The listing builds one solid part. Answer for the finished solid, in the listing's coordinates (mm). Face numbers are marked on the shaded views. A direction names the side the tool comes from. Round coordinates to 2 decimals unless told otherwise and drop trailing zeros. Write each loop counter-clockwise with the first axis right and the second up, starting at its lowest first coordinate (ties: lowest second). Pieces come first, ordered by that corner, then holes. Notation, with made-up numbers: (65.25, -25) - (124.25, -25) arc R25 ccw to (124.25, 14) - close; hole circle Ø4 at (25.25, -28.5). An arc over 180 degrees is marked (long way). Use a Markdown table: item, result. Add a question column.
1) Determine the mould class of the marked faces 1, 2, 3 and 4 for opening direction X: +X half, -X half, draft (parallel to the pull), parting line (faces both ways), or undercut.
2) Find the intervals of material crossed by probe 1 along X at (y, z) = (15.25, 0); probe 2 along X at (y, z) = (21, -7.5); probe 3 along Z at (x, y) = (-8.5, 3.25), in increasing order. Write a range as from..to.
3) A cutting plane is placed at B-B (y = 11). Give the vertices of the cut face in (x, z), then the cut area to 3 significant figures.
4) A cutting plane is placed at D-D (x = 0). Give the vertices of the cut face in (y, z), then the cut area to 3 significant figures.
5) A cutting plane is placed at A-A (x = -15.05). Give the vertices of the cut face in (y, z).
6) Each of these flat-tipped pins is pushed along its axis until it touches: P1, Ø2, axis at x = 19.5, y = 6, coming from the -Z side; P2, Ø3.5, axis at y = 5, z = -18, coming from the +X side; P3, Ø4, axis at x = 43.53, z = -15, coming from the +Y side. Where does it stop, or does it pass through?
7) A tool of negligible diameter and unlimited length cuts with its end or side. For the marked faces 5, 6 and 7, from which of +Z, -Z, +X, -X, +Y, -Y can it reach the whole face along a straight path? Write none if from no direction.
8) A cutting plane is placed at C-C (y = 6). Give the vertices of the cut face in (x, z).
```python
from build123d import *

# Parameters (mm, degrees)
BOSS_EXTRUDE1_DEPTH             = 25
SKETCH2_R                       = 1.55
CUT_EXTRUDE1_DEPTH              = 22.5
BOSS_EXTRUDE2_REACH             = 65.436
BOSS_EXTRUDE2_DIRECTION_2_DEPTH = 30
CUT_EXTRUDE2_REACH              = 80.642
CUT_EXTRUDE2_END_RADIUS         = 17.5
SKETCH7_R                       = 1.55
SKETCH9_R                       = 2.05
CUT_EXTRUDE3_DEPTH              = 35.1
BOSS_EXTRUDE5_REACH             = 63.632


with BuildPart() as part:
    # Sketch1 → Boss-Extrude1 (new, symmetric)
    with BuildSketch(Plane.XY):
        with BuildLine():
            Line((-17.55, 22.5), (-17.55, 0))
            Line((-17.55, 0), (17.55, 0))
            Line((17.55, 0), (17.55, 22.5))
            Line((17.55, 22.5), (12.55, 22.5))
            ThreePointArc((12.55, 22.5), (0, 9.95), (-12.55, 22.5))
            Line((-12.55, 22.5), (-17.55, 22.5))
        make_face()
    extrude(amount=BOSS_EXTRUDE1_DEPTH, both=True)

    # Sketch2 → Cut-Extrude1 (cut)
    with BuildSketch(Plane(origin=(0, 22.5, 0), x_dir=(1, 0, 0), z_dir=(0, 1, 0))):
        with Locations(Location((-15.05, 0, 0), (0, 0, 270))):
            Circle(SKETCH2_R)
        with Locations(Location((15.05, 0, 0), (0, 0, 270))):
            Circle(SKETCH2_R)
    extrude(amount=-CUT_EXTRUDE1_DEPTH, mode=Mode.SUBTRACT)

    # Boss-Extrude2: up to this plane
    boss_extrude2_end = Plane(origin=(17.55, 0, 25), z_dir=(-1, 0, 0))
    # Sketch5 → Boss-Extrude2 (add, up to the surface)
    with BuildSketch(Plane(origin=(26.152881057, 0, -15.099372918), x_dir=(-0.5000000000000013, 0, -0.8660254037844379), z_dir=(0.8660254037844379, 0, -0.5000000000000013)), mode=Mode.PRIVATE) as boss_extrude2_sk1:
        with BuildLine():
            Line((-26.275, 22.5), (-21.325, 22.5))
            ThreePointArc((-21.325, 22.5), (-8.775, 9.95), (3.775, 22.5))
            Line((3.775, 22.5), (8.725, 22.5))
            ThreePointArc((8.725, 22.5), (-8.775, 5), (-26.275, 22.5))
        make_face()
    boss_extrude2_tool1 = split(extrude(boss_extrude2_sk1.sketch, amount=-BOSS_EXTRUDE2_REACH, mode=Mode.PRIVATE), bisect_by=boss_extrude2_end, keep=Keep.BOTH, mode=Mode.PRIVATE)
    add(boss_extrude2_tool1.solids().sort_by_distance((38.052881, 22.108688, 5.512032))[0])

    # Sketch5 → Boss-Extrude2 direction 2 (add)
    with BuildSketch(Plane(origin=(26.152881057, 0, -15.099372918), x_dir=(-0.5000000000000013, 0, -0.8660254037844379), z_dir=(0.8660254037844379, 0, -0.5000000000000013))):
        with BuildLine():
            Line((-26.275, 22.5), (-21.325, 22.5))
            ThreePointArc((-21.325, 22.5), (-8.775, 9.95), (3.775, 22.5))
            Line((3.775, 22.5), (8.725, 22.5))
            ThreePointArc((8.725, 22.5), (-8.775, 5), (-26.275, 22.5))
        make_face()
    extrude(amount=BOSS_EXTRUDE2_DIRECTION_2_DEPTH)

    # Cut-Extrude2: up to this cylinder (the profile starts inside it)
    cut_extrude2_end = Plane(origin=(43.530762028, 22.5, -14.999999951), z_dir=(-0.8660254037844379, 0, 0.5000000000000013)) * Cylinder(CUT_EXTRUDE2_END_RADIUS, 197.284, mode=Mode.PRIVATE)
    # Sketch7 → Cut-Extrude2 (cut, up to the surface)
    with BuildSketch(Plane(origin=(0, 22.5, 0), x_dir=(1, 0, 0), z_dir=(0, 1, 0)), mode=Mode.PRIVATE) as cut_extrude2_sk1:
        with Locations(Location((43.530762114, 15, 0), (0, 0, 180))):
            Circle(SKETCH7_R)
    cut_extrude2_tool1 = extrude(cut_extrude2_sk1.sketch, amount=-CUT_EXTRUDE2_REACH, mode=Mode.PRIVATE) & cut_extrude2_end
    add(cut_extrude2_tool1.solids().sort_by_distance((43.530762, 22.5, -15))[0], mode=Mode.SUBTRACT)

    # Sketch9 → Cut-Extrude3 (cut)
    with BuildSketch(Plane.ZY.offset(17.55)):
        with Locations((-18, 5)):
            Circle(SKETCH9_R)
        with Locations((18, 5)):
            Circle(SKETCH9_R)
    extrude(amount=-CUT_EXTRUDE3_DEPTH, mode=Mode.SUBTRACT)

    # Boss-Extrude5: up to this face of the body (flat: up to its plane)
    boss_extrude5_end = Plane(part.part.faces().sort_by_distance((17.55, 17.173614571, 0))[0])
    # Sketch12 → Boss-Extrude5 (add, up to the picked face)
    with BuildSketch(Plane(origin=(22.035576211, 0, -12.722245857), x_dir=(-0.4999999999999781, 0, -0.8660254037844513), z_dir=(0.8660254037844513, 0, -0.4999999999999781)), mode=Mode.PRIVATE) as boss_extrude5_sk1:
        with BuildLine():
            Line((-21.325, 22.5), (3.775, 22.5))
            ThreePointArc((3.775, 22.5), (-8.775, 9.95), (-21.325, 22.5))
        make_face()
    boss_extrude5_tool1 = split(extrude(boss_extrude5_sk1.sketch, amount=-BOSS_EXTRUDE5_REACH, mode=Mode.PRIVATE), bisect_by=boss_extrude5_end, keep=Keep.BOTH, mode=Mode.PRIVATE)
    add(boss_extrude5_tool1.solids().sort_by(Axis((26.423076, 17.173615, -5.122873), (-0.8660254037844513, 0, 0.4999999999999781)))[0])


solid = part.part
```
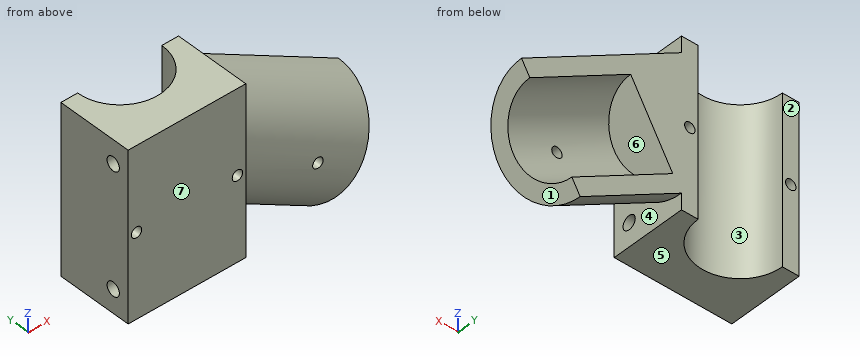
Entries:
| question | item | result |
|---|---|---|
| 1 | face 1 | +X half |
| 1 | face 2 | draft |
| 1 | face 3 | undercut |
| 1 | face 4 | undercut |
| 2 | probe 1 | x = -17.55..-16.6, -13.5..-10.24, 10.24..13.5, 16.6..29.38, 38.04..49.41 |
| 2 | probe 2 | x = -17.55..-12.46, 12.46..25.05, 55.46..65.18 |
| 2 | probe 3 | z = -25..-19.07, -16.93..16.93, 19.07..25 |
| 3 | outline | (-17.55, -25) - (-5.03, -25) - (-5.03, 25) - (-17.55, 25) - close; (5.03, -25) - (17.55, -25) - (17.55, -15.23) - (49.93, -33.92) - (54.01, -26.85) - (23.91, -9.47) - (28.94, -0.77) - (59.03, -18.15) - (63.12, -11.08) - (17.55, 15.23) - (17.55, 25) - (5.03, 25) - close; hole circle Ø3.1 at (-15.05, 0); hole circle Ø3.1 at (15.05, 0) |
| 3 | area | 2,080 mm² |
| 4 | outline | (0, -25) - (9.95, -25) - (9.95, 25) - (0, 25) - close; hole circle Ø4.1 at (5, -18); hole circle Ø4.1 at (5, 18) |
| 4 | area | 471 mm² |
| 5 | outline | (0, -25) - (22.5, -25) - (22.5, -1.55) - (0, -1.55) - close; (0, 1.55) - (22.5, 1.55) - (22.5, 25) - (0, 25) - close; hole circle Ø4.1 at (5, -18); hole circle Ø4.1 at (5, 18) |
| 6 | P1 | stops at z = -10.58 |
| 6 | P2 | stops at x = 59.81 |
| 6 | P3 | stops at y = 10.11 |
| 7 | face 5 | -Z, -X, +Y, -Y |
| 7 | face 6 | +Y |
| 7 | face 7 | +Z, -Z, +X, -X, -Y |
| 8 | outline | (-17.55, -25) - (17.55, -25) - (17.55, -19.79) - (-17.55, -19.79) - close; (-17.55, -16.21) - (17.55, -16.21) - (17.55, -6.73) - (53.61, -27.55) - (59.44, -17.45) - (17.55, 6.73) - (17.55, 16.21) - (-17.55, 16.21) - close; (-17.55, 19.79) - (17.55, 19.79) - (17.55, 25) - (-17.55, 25) - close; hole circle Ø3.1 at (-15.05, 0); hole circle Ø3.1 at (15.05, 0); hole circle Ø3.1 at (43.53, -15) |
